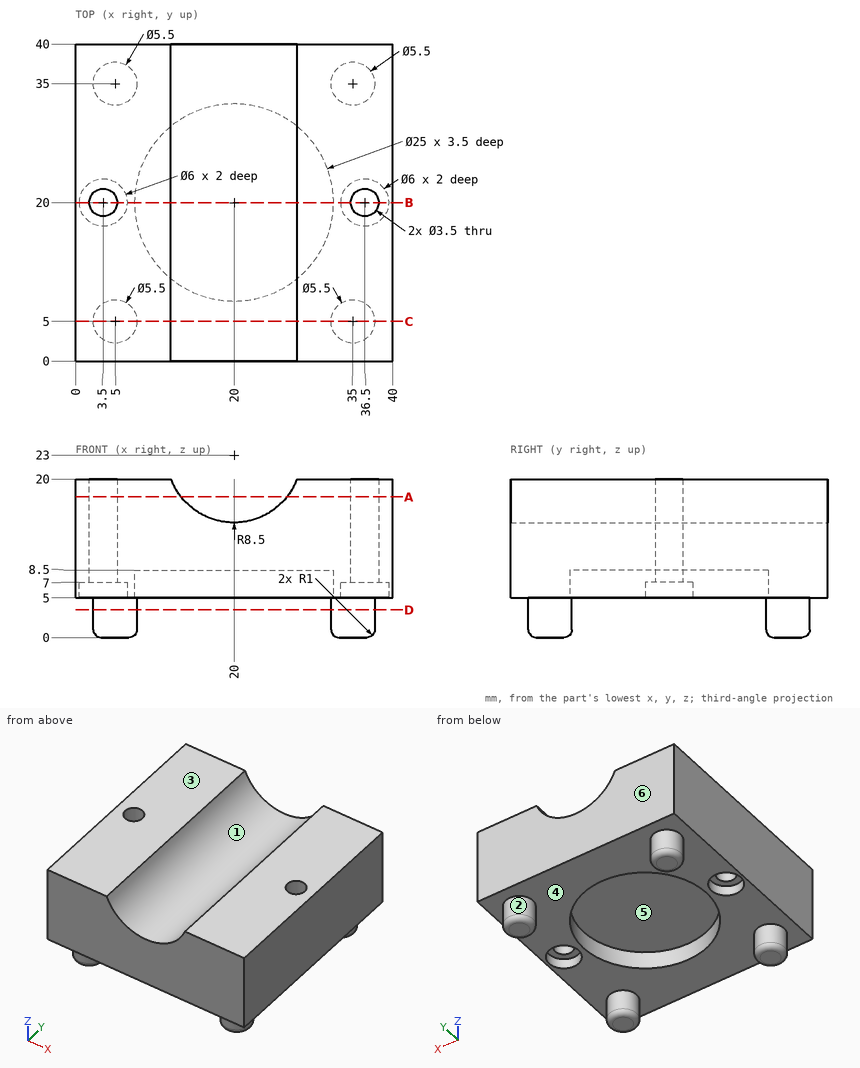
Print and shaded views of the part. All mm, measured from the part's lowest x, y and z. A direction names the side the tool comes from. Give positions to 0.01 mm unless a question says otherwise; leave off trailing zeros. Loops run counter-clockwise (first coordinate to the right, second up) from the corner with the lowest first, then second, coordinate; pieces in that order, holes last. Notation, with made-up numbers: (85.25, 81.25) - (108.25, 81.25) arc R26 ccw to (108.25, 99.25) - close; hole circle Ø10 at (47, 86.25). An arc over 180 degrees is marked (long way). One line per item, written item: value. Start each with the question number.
1. Slice it at C-C (y = 5). List the corners of the cut face in (x, z).
2. Probe L1, parallel to Y at x = 3.5, z = 16.75; L2, parallel to X at y = 21.5, z = 9.75; L3, parallel to Y at x = 36.5, z = 5.75. List the from-to ranges inside material, lowest first. Write a range as from..to.
3. Pin check, flat tips, straight feed: pin 1 (6.5 mm diameter, centred on x = 4, y = 21, fed in from -Z); pin 2 (4.5 mm diameter, centred on x = 3.5, y = 20, fed in from -Z); pin 3 (12.5 mm diameter, centred on x = 20, y = 21.5, fed in from -Z). Stop position of each tip, or through.
4. Slice it at A-A (z = 17.75). List the corners of the cut face in (x, y), plus the area to 3 significant figures.
5. Slice it at D-D (z = 3.5). List the corners of the cut face in (x, y).
6. Slice it at B-B (y = 20). List the corners of the cut face in (x, z), plus the area to 3 significant figures.
7. Pull direction Y, two halves, no side cores. Call the marked faces 3, 4, 5 and 6: pulls with the +Y half, pulls with the -Y half, needs draft (parallel to the pull), parting line crosses it, or undercut.
8. Which spindle directions (+Z, -Z, +X, -X, +Y, -Y) get a long thin tool onto all of the face, cutting with end or side? Do the marked faces 1 and 2. Say none if no direction does.
Solution:
1. outline: (0, 5) - (2.25, 5) - (2.25, 1) arc R1 ccw to (3.25, 0) - (6.75, 0) arc R1 ccw to (7.75, 1) - (7.75, 5) - (32.25, 5) - (32.25, 1) arc R1 ccw to (33.25, 0) - (36.75, 0) arc R1 ccw to (37.75, 1) - (37.75, 5) - (40, 5) - (40, 20) - (27.95, 20) arc R8.5 cw to (12.05, 20) - (0, 20) - close
2. L1: y = 0..18.25, 21.75..40
2. L2: x = 0..2.6, 4.4..35.6, 37.4..40
2. L3: y = 0..17, 23..40
3. pin 1: stops at z = 5
3. pin 2: stops at z = 7
3. pin 3: stops at z = 8.5
4. outline: (0, 0) - (13.32, 0) - (13.32, 40) - (0, 40) - close; (26.68, 0) - (40, 0) - (40, 40) - (26.68, 40) - close; hole circle Ø3.5 at (3.5, 20); hole circle Ø3.5 at (36.5, 20)
4. area: 1,050 mm^2
5. outline: circle Ø5.5 at (5, 5); circle Ø5.5 at (5, 35); circle Ø5.5 at (35, 5); circle Ø5.5 at (35, 35)
6. outline: (0, 5) - (0.5, 5) - (0.5, 7) - (1.75, 7) - (1.75, 20) - (0, 20) - close; (5.25, 7) - (6.5, 7) - (6.5, 5) - (7.5, 5) - (7.5, 8.5) - (32.5, 8.5) - (32.5, 5) - (33.5, 5) - (33.5, 7) - (34.75, 7) - (34.75, 20) - (27.95, 20) arc R8.5 cw to (12.05, 20) - (5.25, 20) - close; (38.25, 7) - (39.5, 7) - (39.5, 5) - (40, 5) - (40, 20) - (38.25, 20) - close
6. area: 334 mm^2
7. face 3: needs draft
7. face 4: undercut
7. face 5: undercut
7. face 6: pulls with the +Y half
8. face 1: +Z, +Y, -Y
8. face 2: -Z
